```python
from build123d import *

# Parameters (mm, degrees)
BOSS_EXTRUDE1_DEPTH = 38.1
SKETCH2_R           = 1.524
CUT_EXTRUDE1_DEPTH  = 57.149295064
SKETCH3_R           = 1.524
CUT_EXTRUDE2_DEPTH  = 45.844943949


with BuildPart() as part:
    # Sketch1 → Boss-Extrude1 (new body)
    with BuildSketch(Plane(origin=(0, 0, 0), x_dir=(0, 0, -1), z_dir=(1, 0, 0))):
        Polygon((-2.180942408, -19.43565445), (15.599057592, -19.43565445), (15.599057592, -37.21565445), (13.059057592, -37.21565445), (13.059057592, -21.97565445), (-2.180942408, -21.97565445), align=None)
    extrude(amount=BOSS_EXTRUDE1_DEPTH)

    # Sketch2 → Cut-Extrude1 (cut, through all)
    with BuildSketch(Plane(origin=(0, 0, -15.599057592), x_dir=(-1, 0, 0), z_dir=(0, 0, -1))):
        with Locations(Location((-34.29, -33.40565445, 0), (0, 0, 90))):
            Circle(SKETCH2_R)
        with Locations(Location((-3.81, -33.40565445, 0), (0, 0, 90))):
            Circle(SKETCH2_R)
        with Locations(Location((-3.81, -27.05565445, 0), (0, 0, 90))):
            Circle(SKETCH2_R)
        with Locations(Location((-34.29, -27.05565445, 0), (0, 0, 90))):
            Circle(SKETCH2_R)
    extrude(amount=-CUT_EXTRUDE1_DEPTH, mode=Mode.SUBTRACT)

    # Sketch3 → Cut-Extrude2 (cut, through all)
    with BuildSketch(Plane(origin=(0, -19.43565445, 0), x_dir=(1, 0, 0), z_dir=(0, 1, 0))):
        with Locations(Location((3.81, 1.629057592, 0), (0, 0, 270))):
            Circle(SKETCH3_R)
        with Locations(Location((34.29, 1.629057592, 0), (0, 0, 270))):
            Circle(SKETCH3_R)
        with Locations(Location((3.81, 7.979057592, 0), (0, 0, 270))):
            Circle(SKETCH3_R)
        with Locations(Location((34.29, 7.979057592, 0), (0, 0, 270))):
            Circle(SKETCH3_R)
    extrude(amount=-CUT_EXTRUDE2_DEPTH, mode=Mode.SUBTRACT)


solid = part.part
```
CAD build for the part. Positions are in the model's coordinates, mm. A direction names the side the tool comes from. Round coordinates to 2 decimals unless told otherwise and drop trailing zeros. Write each loop counter-clockwise with the first axis right and the second up, starting at its lowest first coordinate (ties: lowest second). Pieces come first, ordered by that corner, then holes. Notation, with made-up numbers: (-23, 86.25) - (-4, 86.25) arc R14 cw to (-4, 101.25) - close; hole circle Ø7 at (-25, 48.25). An arc over 180 degrees is marked (long way). Return JSON: item names as keys, results as strings. Group by question number.
Item 1: Band-saw the part on A-A on x = 34.29. List the corners of the cut face in (y, z).
Item 2: 3-axis set-ups, long thin cutter, end or side, ignore diameter. For faces 5 (the face through (19, -30, -13.059)), 6 (the face through (35.8, -27.25, -14.35)): which of +Z, -Z, +X, -X, +Y, -Y reach the whole face in a straight line?
Item 3: Flat gauge pins, fed straight in: pin 1 Ø4 at (x, y) = (34.29, -27.06) entering from +Z; pin 2 Ø2 at (x, z) = (32.5, -10.5) entering from -Y; pin 3 Ø2.5 at (x, y) = (34.29, -33.41) entering from -Z. Where does each tip first touch, or does it go through?
Item 4: Mould opens along Y. For faces 1 (the face through (19, -21.976, -6)), 2 (the face through (19, -19.436, -7)), 3 (the face through (4.268, -20.688, -6.525)), 4 (the face through (4.268, -31.952, -14.347)) say: +Y half, -Y half, draft (parallel to the pull), parting line (faces both ways), or undercut.
Item 5: Band-saw the part on B-B on y = -20.25. List the corners of the cut face in (x, z).
Item 6: Band-saw the part on D-D on y = -34.5. List the corners of the cut face in (x, z), plus the area to 3 significant figures.
Item 7: Probe probe 1 along Z at (x, y) = (15.5, -24); probe 2 along Y at (x, z) = (4, -11.5). List the from-to ranges inside material, lowest first.
Item 8: Band-saw the part on C-C on z = -13.75. List the corners of the cut face in (x, y), plus the area to 3 significant figures.
Resolved:
{
 "1": {"outline": "(-37.22, -15.6) - (-34.93, -15.6) - (-34.93, -13.06) - (-37.22, -13.06) - close; (-31.88, -15.6) - (-28.58, -15.6) - (-28.58, -13.06) - (-31.88, -13.06) - close; (-25.53, -15.6) - (-19.44, -15.6) - (-19.44, -9.5) - (-21.98, -9.5) - (-21.98, -13.06) - (-25.53, -13.06) - close; (-21.98, -6.46) - (-19.44, -6.46) - (-19.44, -3.15) - (-21.98, -3.15) - close; (-21.98, -0.11) - (-19.44, -0.11) - (-19.44, 2.18) - (-21.98, 2.18) - close"},
 "2": {"face 5": "+Z, +X, -X, -Y", "face 6": "+Z, -Z"},
 "3": {"pin 1": "stops at z = -13.06", "pin 2": "stops at y = -21.98", "pin 3": "passes through"},
 "4": {"face 1": "-Y half", "face 2": "+Y half", "face 3": "draft", "face 4": "undercut"},
 "5": {"outline": "(0, -15.6) - (38.1, -15.6) - (38.1, 2.18) - (0, 2.18) - close; hole circle Ø3.05 at (3.81, -7.98); hole circle Ø3.05 at (3.81, -1.63); hole circle Ø3.05 at (34.29, -7.98); hole circle Ø3.05 at (34.29, -1.63)"},
 "6": {"outline": "(0, -15.6) - (2.75, -15.6) - (2.75, -13.06) - (0, -13.06) - close; (4.87, -15.6) - (33.23, -15.6) - (33.23, -13.06) - (4.87, -13.06) - close; (35.35, -15.6) - (38.1, -15.6) - (38.1, -13.06) - (35.35, -13.06) - close", "area": "86.0 mm²"},
 "7": {"probe 1": "z = -15.6 to -13.06", "probe 2": "y = -21.98 to -19.44"},
 "8": {"outline": "(0, -37.22) - (38.1, -37.22) - (38.1, -19.44) - (0, -19.44) - close; hole circle Ø3.05 at (3.81, -33.41); hole circle Ø3.05 at (3.81, -27.06); hole circle Ø3.05 at (34.29, -33.41); hole circle Ø3.05 at (34.29, -27.06)", "area": "648 mm²"}
}
